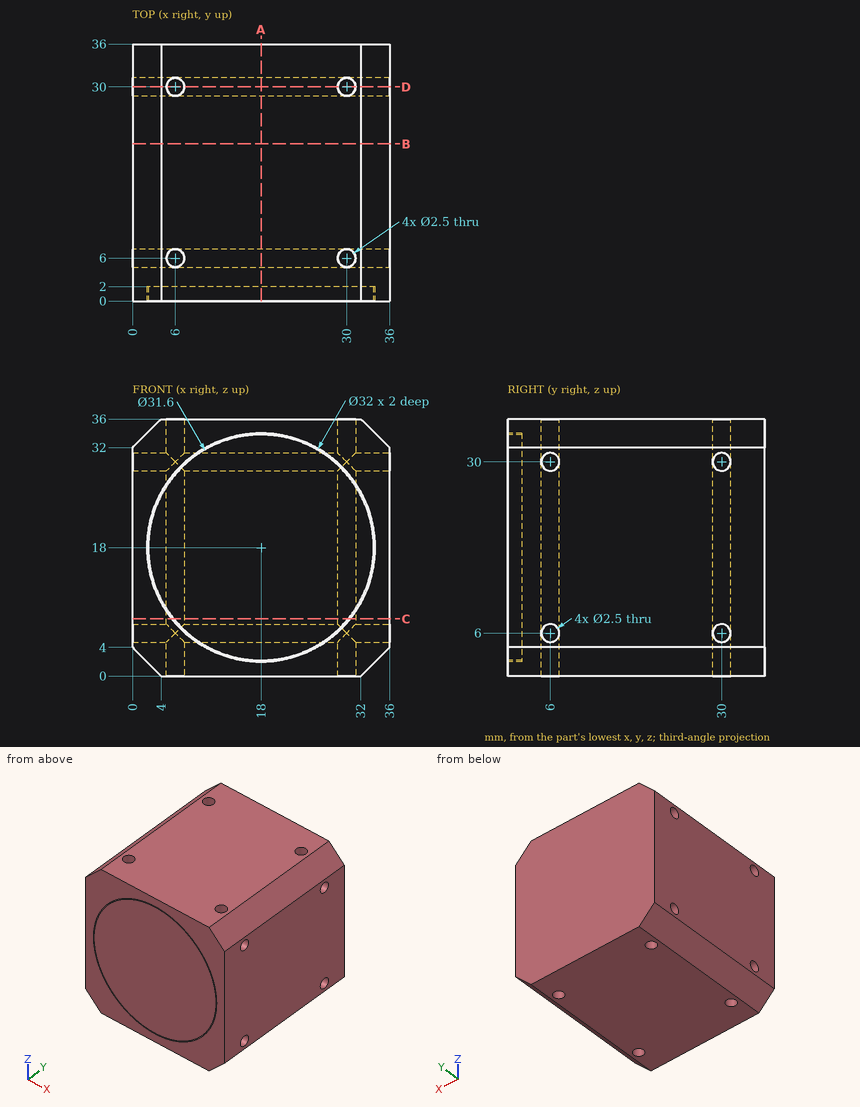
Answer from the drawing. Dimensions are ordinates in mm from the lowest x, y and z of the part. Give positions to 0.01 mm unless a question says otherwise; leave off trailing zeros. Write each loop counter-clockwise with the first axis right and the second up, starting at its lowest first coordinate (ties: lowest second). Pieces come first, ordered by that corner, then holes. Notation, with made-up numbers: (86, -36.5) - (122, -36.5) arc R19 ccw to (122, -21.5) - close; hole circle Ø6 at (16.5, -39). An arc over 180 degrees is marked (long way). One line per item, written item: value. Start each with the question number.
1. Find section D-D (y = 30). State how many separate pieces and enclosed holes the cut face has, then the cut area to 3 significant figures.
2. Consider probe 1 along Y at (x, z) = (20.5, 30); probe 2 along Y at (x, z) = (4, 6.5). Determine where each line is inside the solid, lowest interval first.
3. Find section C-C (z = 8). Write down the section's boundary in (x, y), then the cut area to 3 significant figures.
4. Find section B-B (y = 22). Write down the section's boundary in (x, z), then the cut area to 3 significant figures.
5. Find section A-A (x = 18). Write down the section's boundary in (y, z).
Geometry results:
1. separate pieces: 9
1. enclosed holes: 0
1. area: 929 mm2
2. probe 1: 0 to 4.75, 7.25 to 28.75, 31.25 to 36
2. probe 2: 0 to 4.85, 7.15 to 28.85, 31.15 to 36
3. outline: (0, 0) - (5.51, 0) - (5.51, 2) - (5.77, 2) - (5.77, 0) - (30.23, 0) - (30.23, 2) - (30.49, 2) - (30.49, 0) - (36, 0) - (36, 36) - (0, 36) - close; hole circle Ø2.5 at (6, 6); hole circle Ø2.5 at (6, 30); hole circle Ø2.5 at (30, 6); hole circle Ø2.5 at (30, 30)
3. area: 1,280 mm2
4. outline: (0, 4) - (4, 0) - (32, 0) - (36, 4) - (36, 32) - (32, 36) - (4, 36) - (0, 32) - close
4. area: 1,260 mm2
5. outline: (0, 0) - (36, 0) - (36, 36) - (0, 36) - (0, 34) - (2, 34) - (2, 33.8) - (0, 33.8) - (0, 2.2) - (2, 2.2) - (2, 2) - (0, 2) - close; hole circle Ø2.5 at (6, 6); hole circle Ø2.5 at (6, 30); hole circle Ø2.5 at (30, 6); hole circle Ø2.5 at (30, 30)
